CAD build for the part. Positions are in the model's coordinates, mm. A direction names the side the tool comes from. Round coordinates to 2 decimals unless told otherwise and drop trailing zeros. Loops run counter-clockwise (first coordinate to the right, second up) from the corner with the lowest first, then second, coordinate; pieces in that order, holes last.
from build123d import *

# Parameters (mm, degrees)
EXTRUDE_1_DEPTH = 1
EXTRUDE_2_DEPTH = 12.5
EXTRUDE_4_DEPTH = 1


with BuildPart() as part:
    # 草图1 → 凸台-拉伸1 (new body)
    with BuildSketch(Plane.XY):
        Polygon((-53.921953221, 26.960976611), (-53.921953221, 20.960976611), (-36.921953221, 20.960976611), (-36.921953221, 15.960976611), (-28.921953221, 15.960976611), (-28.921953221, 26.960976611), align=None)
    extrude(amount=EXTRUDE_1_DEPTH)

    # 草图2 → 凸台-拉伸2 (add)
    with BuildSketch(Plane.XY.offset(1)):
        Polygon((-53.921953221, 26.960976611), (-52.921953221, 26.960976611), (-52.921953221, 21.960976611), (-35.921953221, 21.960976611), (-35.921953221, 16.960976611), (-29.921953221, 16.960976611), (-29.921953221, 26.960976611), (-28.921953221, 26.960976611), (-28.921953221, 15.960976611), (-36.921953221, 15.960976611), (-36.921953221, 20.960976611), (-53.921953221, 20.960976611), align=None)
    extrude(amount=EXTRUDE_2_DEPTH)

    # 草图4 → 凸台-拉伸4 (add)
    with BuildSketch(Plane.XY.offset(13.5)):
        Polygon((-53.921953221, 26.960976611), (-28.921953221, 26.960976611), (-28.921953221, 15.960976611), (-36.921953221, 15.960976611), (-36.921953221, 20.960976611), (-53.921953221, 20.960976611), align=None)
    extrude(amount=EXTRUDE_4_DEPTH)


solid = part.part
Item 1: 3-axis set-ups, long thin cutter, end or side, ignore diameter. For faces 4 (the flat face through (-53.922, 24, 7)), 5 (the flat face through (-45, 20.961, 7)), 6 (the flat face through (-39, 23, 13.5)): which of +Z, -Z, +X, -X, +Y, -Y reach the whole face in a straight line?
Verdict:
face 4: +Z, -Z, -X, +Y, -Y
face 5: +Z, -Z, -X, -Y
face 6: +Y
Item 2: Cut at D-D (y = 18.25). List the corners of the cut face in (x, z).
Verdict:
outline: (-36.92, 0) - (-28.92, 0) - (-28.92, 14.5) - (-36.92, 14.5) - close; hole (-35.92, 1) - (-29.92, 1) - (-29.92, 13.5) - (-35.92, 13.5) - close
Item 3: Flat gauge pins, fed straight in: P1, Ø4, axis at x = -42, z = 8.5, coming from the +Y side; P2, Ø4, axis at y = 18.5, z = 9, coming from the -X side; P3, Ø3, axis at x = -33, z = 7, coming from the +Y side; P4, Ø5, axis at x = -39, y = 20, coming from the +Z side. Where does each tip first touch, or does it go through?
Verdict:
P1: stops at y = 21.96
P2: stops at x = -36.92
P3: stops at y = 16.96
P4: stops at z = 14.5
Item 4: Cut at B-B (x = -36.5). List the corners of the cut face in (y, z).
Verdict:
outline: (15.96, 0) - (26.96, 0) - (26.96, 1) - (21.96, 1) - (21.96, 13.5) - (26.96, 13.5) - (26.96, 14.5) - (15.96, 14.5) - close
Item 5: Mould opens along X. For faces 1 (the flat face through (-39, 23, 1)), 2 (the flat face through (-36.922, 18, 7)), 3 (the flat face through (-38, 23, 14.5)) say: released by +X, released by -X, zero draft, split by the parting line, or undercut.
Verdict:
face 1: undercut
face 2: released by -X
face 3: zero draft
Item 6: Cut at A-A (y = 21.5). List the corners of the cut face in (x, z), plus the area to 4 significant figures.
Verdict:
outline: (-53.92, 0) - (-28.92, 0) - (-28.92, 14.5) - (-53.92, 14.5) - close; hole (-35.92, 1) - (-29.92, 1) - (-29.92, 13.5) - (-35.92, 13.5) - close
area: 287.5 mm2
Item 7: Wall check: L1, parallel to Z at x = -30.25, y = 17; L2, parallel to X at y = 23.5, z = 6.25; L3, parallel to X at y = 20.5, z = 10. Give the ranges that are in metal, low to high.
Verdict:
L1: z = 0 to 1, 13.5 to 14.5
L2: x = -53.92 to -52.92, -29.92 to -28.92
L3: x = -36.92 to -35.92, -29.92 to -28.92
Item 8: Cut at C-C (z = 2.25). List the corners of the cut face in (x, y).
Verdict:
outline: (-53.92, 20.96) - (-36.92, 20.96) - (-36.92, 15.96) - (-28.92, 15.96) - (-28.92, 26.96) - (-29.92, 26.96) - (-29.92, 16.96) - (-35.92, 16.96) - (-35.92, 21.96) - (-52.92, 21.96) - (-52.92, 26.96) - (-53.92, 26.96) - close
